Answer from the drawing. Dimensions are ordinates in mm from the lowest x, y and z of the part. A direction names the side the tool comes from. Give positions to 0.01 mm unless a question says otherwise; leave off trailing zeros. Loops run counter-clockwise (first coordinate to the right, second up) from the corner with the lowest first, then second, coordinate; pieces in that order, holes last.
Item 1: A tool of negligible diameter and unlimited length cuts with its end or side. For the marked faces 5, 6 and 7, from which of +Z, -Z, +X, -X, +Y, -Y can it reach the whole face along a straight path? Write none if from no direction.
Item 2: The mould has two halves that part along X. Classify the marked faces 1, 2, 3 and 4: pulls with the +X half, pulls with the -X half, needs draft (parallel to the pull), parting line crosses it, or undercut.
Item 3: Section A-A, the plane y = 41.5 is taken. Give the vertices of the cut face in (x, z), and give its area (3 significant figures).
Item 4: Section B-B, the plane x = 6.5 is taken. Give the vertices of the cut face in (y, z), and give its area (3 significant figures).
Item 5: Each of these flat-tipped pins is pushed along its axis until it touches: pin 1 Ø1.5 at (x, z) = (11.5, 11) entering from -Y; pin 2 Ø6 at (y, z) = (26, 5) entering from -X; pin 3 Ø3.5 at (y, z) = (5, 10) entering from +X. Where does it stop, or does it pass through?
Item 6: Section C-C, the plane z = 10 is taken. Give the vertices of the cut face in (x, y).
Item 7: Section D-D, the plane y = 5 is taken. Give the vertices of the cut face in (x, z), and give its area (3 significant figures).
Item 8: Consider line 1 along Z through (x, y) = (2.25, 5); line 2 along X through (y, z) = (23.5, 6.5); line 3 along Y through (x, z) = (5.5, 10.25). Determine where each line is inside the solid, lowest interval first.
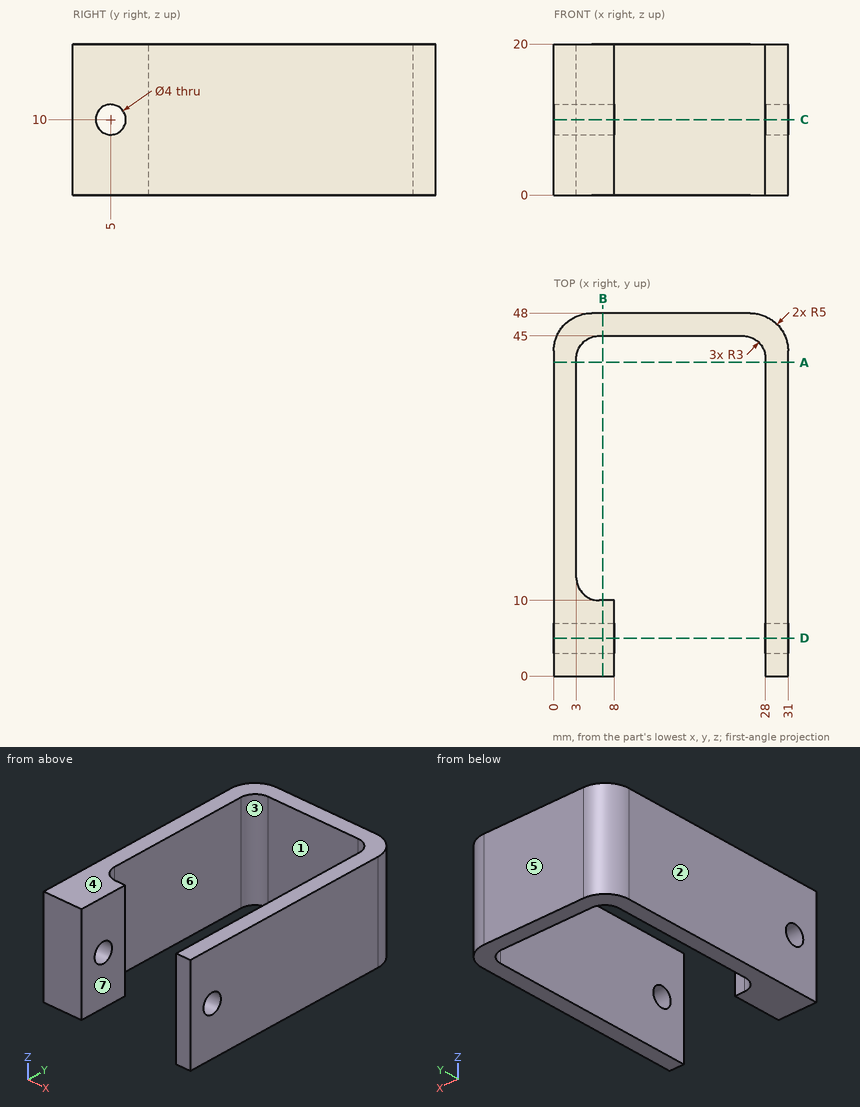
Worked answers:
1. face 5: +Z, -Z, +X, -X, +Y
1. face 6: +Z, -Z
1. face 7: +Z, -Z, -Y
2. face 1: undercut
2. face 2: pulls with the -X half
2. face 3: undercut
2. face 4: needs draft
3. outline: (0, 0) - (3, 0) - (3, 20) - (0, 20) - close; (28, 0) - (31, 0) - (31, 20) - (28, 20) - close
3. area: 120 mm2
4. outline: (0, 0) - (10, 0) - (10, 20) - (0, 20) - close; (45, 0) - (48, 0) - (48, 20) - (45, 20) - close; hole circle Ø4 at (5, 10)
4. area: 247 mm2
5. pin 1: stops at y = 45
5. pin 2: stops at x = 0
5. pin 3: passes through
6. outline: (0, 0) - (8, 0) - (8, 3) - (0, 3) - close; (0, 7) - (8, 7) - (8, 10) - (6, 10) arc R3 cw to (3, 13) - (3, 42) arc R3 cw to (6, 45) - (25, 45) arc R3 cw to (28, 42) - (28, 7) - (31, 7) - (31, 43) arc R5 ccw to (26, 48) - (5, 48) arc R5 ccw to (0, 43) - close; (28, 0) - (31, 0) - (31, 3) - (28, 3) - close
7. outline: (0, 0) - (8, 0) - (8, 8) - (0, 8) - close; (0, 12) - (8, 12) - (8, 20) - (0, 20) - close; (28, 0) - (31, 0) - (31, 8) - (28, 8) - close; (28, 12) - (31, 12) - (31, 20) - (28, 20) - close
7. area: 176 mm2
8. line 1: z = 0 to 8, 12 to 20
8. line 2: x = 0 to 3, 28 to 31
8. line 3: y = 0 to 3.02, 6.98 to 10.04, 44.96 to 48
